Build history of the part. All positions in model axes, mm. Give positions to 0.01 mm unless a question says otherwise; leave off trailing zeros. Write each loop counter-clockwise with the first axis right and the second up, starting at its lowest first coordinate (ties: lowest second). Pieces come first, ordered by that corner, then holes. Notation, with made-up numbers: (41, 9) -> (85, 9) arc R15 ccw to (85, 13) -> close; hole circle Ø2 at (87.25, 81). An arc over 180 degrees is marked (long way). Write item = value, one per line. Start each with the question number.
Q1. Mould opens along Z. For faces 1 (the face through (0.7, -1.2, 4)), 2 (the face through (0.74, -0.772, 101.066)), 3 (the face through (1.5, 0, 50)) say: pulls with the +Z half, pulls with the -Z half, needs draft (parallel to the pull), parting line crosses it, or undercut.
Q2. Drop a flat-ended pin along its axis: P1, Ø1.1, axis at y = -0.25, z = 99.93, coming from the -X side. Give the stop position or say it passes through.
Q3. Wall check: line 1 (Z direction, x = 1.3, y = -4.5); line 2 (Y direction, x = 0.65, z = 66.5); line 3 (Y direction, x = 0.7, z = 0). Give the ranges that are in metal, low to high.
Q4. Saw through at B-B, the plane z = 30.5. List the corners of the cut face in (x, y).
Q5. Saw through at A-A, the plane x = 1. List the corners of the cut face in (y, z), then the cut area to 3 significant figures.
from build123d import *

# Parameters (mm, degrees)
SCHIZZO2_R                   = 0.6
SCHIZZO2_R_2                 = 0.75
ESTRUSIONE_ESTRUSIONE1_DEPTH = 1.5


with BuildPart() as part:
    # Schizzo2 → Estrusione-Estrusione1 (new body)
    with BuildSketch(Plane(origin=(0, 0, 0), x_dir=(0, 0, -1), z_dir=(1, 0, 0))):
        with BuildLine():
            Line((-8.332291626, 0.388194417), (0.430512151, -2.826475698))
            ThreePointArc((0.430512151, -2.826475698), (0.910624595, -4.856307682), (-1.144864856, -4.501781289))
            ThreePointArc((-1.144864856, -4.501781289), (-1.606556333, -3.847632001), (-2.287829183, -3.426992469))
            Line((-2.287829183, -3.426992469), (-8.598749951, -1.111805583))
            ThreePointArc((-8.598749951, -1.111805583), (-10.293839466, -0.654139343), (-12.04284716, -0.5))
            Line((-12.04284716, -0.5), (-97.584454883, -0.5))
            ThreePointArc((-97.584454883, -0.5), (-98.368919424, -0.660267578), (-99.027659733, -1.115384615))
            ThreePointArc((-99.027659733, -1.115384615), (-101.079495527, -0.740290338), (-99.929662763, 1))
            Line((-99.929662763, 1), (-11.776388835, 1))
            ThreePointArc((-11.776388835, 1), (-10.027381141, 0.845860657), (-8.332291626, 0.388194417))
        make_face()
        with Locations((-99.929662763, -0.25)):
            Circle(SCHIZZO2_R, mode=Mode.SUBTRACT)
        with Locations((0, -4)):
            Circle(SCHIZZO2_R_2, mode=Mode.SUBTRACT)
    extrude(amount=ESTRUSIONE_ESTRUSIONE1_DEPTH)


solid = part.part
Report:
q1.face_1 = pulls with the -Z half
q1.face_2 = undercut
q1.face_3 = needs draft
q2.P1 = through
q3.line_1 = -1.15 to -0.56, 0.56 to 1.15
q3.line_2 = -0.5 to 1
q3.line_3 = -5.25 to -4.75, -3.25 to -2.67
q4.outline = (0, -0.5) -> (1.5, -0.5) -> (1.5, 1) -> (0, 1) -> close
q5.outline = (-4.5, 1.14) arc R1.25 ccw (long way) to (-2.83, -0.43) -> (0.39, 8.33) arc R10 ccw to (1, 11.78) -> (1, 99.93) arc R1.25 ccw (long way) to (-1.12, 99.03) arc R2 cw to (-0.5, 97.58) -> (-0.5, 12.04) arc R10 cw to (-1.11, 8.6) -> (-3.43, 2.29) arc R2 cw to start; hole circle Ø1.5 at (-4, 0); hole circle Ø1.2 at (-0.25, 99.93)
q5.area = 155 mm2
